Design review of the part built by this model. Coordinates are the model's own, in mm. Face numbers are marked on the shaded views. A direction names the side the tool comes from. Round coordinates to 2 decimals unless told otherwise and drop trailing zeros. Write item = value, one per line. Start each with the question number.
Item 1: Add section A-A, the plane x = 56. State how many separate pieces and enclosed holes the cut face has, then the cut area to 3 significant figures.
Item 2: For pin 1 Ø1 at (x, y) = (-46.5, 58) entering from +Z; pin 2 Ø1.5 at (x, z) = (-59.5, 37.5) entering from +Y; pin 3 Ø1.5 at (x, y) = (22, 33.5) entering from +Z; pin 4 Ø10 at (x, z) = (-12, -47) entering from +Y, all flat-tipped, find the tip position at first contact; note any pin that passes through.
Item 3: Machinability: for the marked faces 5 and 6, which of the approach directions +Z, -Z, +X, -X, +Y, -Y give a long, thin tool a straight path to every point of the face, cutting with its end or side? Answer none if there is none.
Item 4: To check wall thickness, follow L1, parallel to Y at x = 44, z = -19; L2, parallel to Z at x = -21.5, y = 62; L3, parallel to Z at x = -14, y = 57. State the ranges of each line that lie inside material, in increasing order.
Item 5: Mouldability with a two-part tool opening along Z and no side actions: class the marked faces 1, 2, 3 and 4 as released by +Z, released by -Z, zero draft, split by the parting line, or undercut.
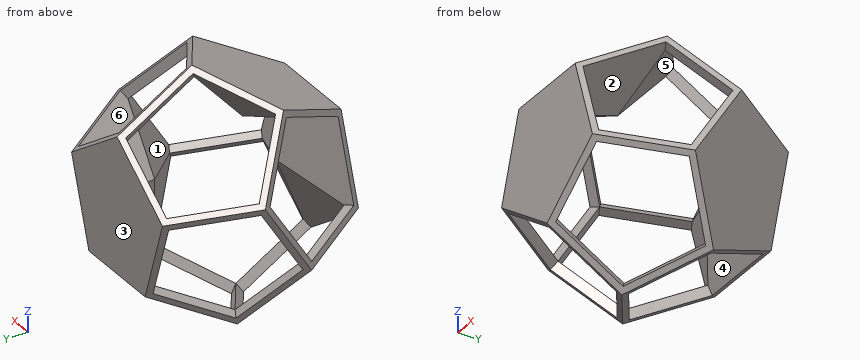
from build123d import *

# Parameters (mm, degrees)
CREATION_EXTRUDE_DEPTH = 130.901699304
CREATION_EXTRUDE_TAPER = -26.56505118
SKETCH2_OUTSIDE_W      = 455.432
SKETCH2_OUTSIDE_H      = 443.246
CREATION_CUT_DEPTH     = 130.901699304
CREATION_CUT_TAPER     = 26.56505118
CUT_EXTRUDE_B_DEPTH    = 50.8
C_INV_DEPTH            = 50.8
CUT_EXTRUDE_D_DEPTH    = 50.8
D_INV_DEPTH            = 50.8
CUT_EXTRUDE_E_DEPTH    = 50.8
E_INV_DEPTH            = 50.8
CUT_EXTRUDE_F_DEPTH    = 50.8
F_INV_DEPTH            = 50.8


with BuildPart() as part:
    # Sketch1 → creation_extrude (new body)
    with BuildSketch(Plane(origin=(0, 0, 0), x_dir=(1, 0, 0), z_dir=(0, 1, 0))):
        Polygon((0, 49.999999949), (-47.552825766, 15.450849703), (-29.389262585, -40.450849677), (29.389262585, -40.450849677), (47.552825766, 15.450849703), align=None)
    extrude(amount=CREATION_EXTRUDE_DEPTH, taper=CREATION_EXTRUDE_TAPER)

    # Sketch2 outside → creation_cut (cut)
    with BuildSketch(Plane(origin=(0, 130.901699304, 0), x_dir=(1, 0, 0), z_dir=(0, 1, 0))):
        with Locations((0, 12.5)):
            Rectangle(SKETCH2_OUTSIDE_W, SKETCH2_OUTSIDE_H)
        Polygon((0, -49.999999949), (47.552825766, -15.450849703), (29.389262585, 40.450849677), (-29.389262585, 40.450849677), (-47.552825766, -15.450849703), align=None, mode=Mode.SUBTRACT)
    extrude(amount=-CREATION_CUT_DEPTH, taper=CREATION_CUT_TAPER, mode=Mode.SUBTRACT)

    # Sketch5 → Cut-Extrude B (cut)
    with BuildSketch(Plane(origin=(0, 42.360679738, -84.721359466), x_dir=(-1, 0, 0), z_dir=(-9.08060963965006e-15, 0.4472135955455734, -0.8944271909771081))):
        Polygon((-42.797543189, 44.635254864), (1e-09, 13.541019643), (42.79754319, 44.635254866), (26.450336325, 94.946784308), (-26.450336327, 94.946784307), align=None)
    extrude(amount=-CUT_EXTRUDE_B_DEPTH, mode=Mode.SUBTRACT)

    # Sketch8 → C_inv (cut)
    with BuildSketch(Plane(origin=(-30.776835339, -16.180339872, 9.999999989), x_dir=(0.2446443083020028, 0.12861712429362696, 0.9610446387935747), z_dir=(-0.8506508083303469, -0.4472135955455736, 0.27639320224297786))):
        Polygon((-31.935023341, 77.848060657), (-22.992425992, 25.708717357), (29.358450763, 18.101689683), (52.77047459, 65.539631327), (14.889024305, 102.464919293), align=None)
    extrude(amount=-C_INV_DEPTH, mode=Mode.SUBTRACT)

    # Sketch9 → Cut-Extrude D (cut)
    with BuildSketch(Plane(origin=(49.797965648, 42.360679738, 68.541019594), x_dir=(0.8506508083603209, -0.27639320226847824, -0.44721359547279954), z_dir=(0.5257311121057348, 0.44721359554557366, 0.7236067977315217))):
        Polygon((-4.184405192, 98.473361345), (-54.495934634, 82.126154482), (-54.495934634, 29.22548183), (-4.184405192, 12.878274966), (26.90983003, 55.675818156), align=None)
    extrude(amount=-CUT_EXTRUDE_D_DEPTH, mode=Mode.SUBTRACT)

    # Sketch10 → D_inv (cut)
    with BuildSketch(Plane(origin=(-19.021130306, -16.180339872, -26.180339859), x_dir=(-0.8506508083603233, 0.27639320226847536, 0.44721359547279665), z_dir=(-0.5257311121057309, -0.44721359554557344, -0.7236067977315247))):
        Polygon((31.995934659, 98.473361351), (-18.315594783, 82.126154488), (-18.315594783, 29.225481836), (31.995934659, 12.878274972), (63.090169881, 55.675818162), align=None)
    extrude(amount=-D_INV_DEPTH, mode=Mode.SUBTRACT)

    # Sketch11 → Cut-Extrude E (cut)
    with BuildSketch(Plane(origin=(-49.797965648, 42.360679738, 68.541019594), x_dir=(0.8506508083603298, 0.2763932022684677, 0.447213595472789), z_dir=(-0.5257311121057203, 0.44721359554557355, 0.7236067977315324))):
        Polygon((4.184405192, 98.473361345), (-26.90983003, 55.675818156), (4.184405192, 12.878274966), (54.495934634, 29.22548183), (54.495934634, 82.126154482), align=None)
    extrude(amount=-CUT_EXTRUDE_E_DEPTH, mode=Mode.SUBTRACT)

    # Sketch12 → E_inv (cut)
    with BuildSketch(Plane(origin=(19.021130306, -16.180339872, -26.180339859), x_dir=(-0.8506508083603274, -0.27639320226847064, -0.44721359547279194), z_dir=(0.5257311121057243, -0.44721359554557355, -0.7236067977315294))):
        Polygon((-31.99593466, 98.473361351), (-63.090169881, 55.67581816), (-31.995934658, 12.878274972), (18.315594784, 29.225481837), (18.315594782, 82.126154489), align=None)
    extrude(amount=-E_INV_DEPTH, mode=Mode.SUBTRACT)

    # Sketch13 → Cut-Extrude F (cut)
    with BuildSketch(Plane(origin=(-80.574800989, 42.360679738, -26.180339862), x_dir=(-0.24464430830199108, 0.12861712429362016, 0.9610446387935785), z_dir=(-0.8506508083303513, 0.4472135955455735, -0.2763932022429644))):
        Polygon((-12.522250637, 97.763517637), (-35.934274461, 50.325575991), (1.947175826, 13.400288027), (48.771223471, 38.017146666), (39.828626119, 90.156489966), align=None)
    extrude(amount=-CUT_EXTRUDE_F_DEPTH, mode=Mode.SUBTRACT)

    # Sketch14 → F_inv (cut)
    with BuildSketch(Plane(origin=(30.776835339, -16.180339872, 9.999999989), x_dir=(0.2446443083019939, -0.12861712429362177, -0.9610446387935776), z_dir=(0.8506508083303502, -0.4472135955455736, 0.2763932022429676))):
        Polygon((-29.358450768, 18.101689686), (22.992425988, 25.708717353), (31.935023344, 77.848060652), (-14.889024299, 102.464919294), (-52.770474589, 65.539631333), align=None)
    extrude(amount=-F_INV_DEPTH, mode=Mode.SUBTRACT)


with BuildPart() as body_2:
    # of the pieces the cut leaves, the one that is kept (f_inv_keep)
    add(part.part.solids().sort_by_distance((0, 0, -49.999999949))[0])


solid = body_2.part
Result set:
q1.separate_pieces = 3
q1.enclosed_holes = 0
q1.area = 1,790 mm²
q2.pin_1 = through
q2.pin_2 = 69.71
q2.pin_3 = 57.58
q2.pin_4 = 127.8
q3.face_5 = none
q3.face_6 = +Z
q4.L1 = 1.57 to 4.13, 75.3 to 116.37
q4.L2 = -72.7 to -69.81, 61.99 to 71.45
q4.L3 = -75.06 to -72.39, 53.23 to 68.95
q5.face_1 = undercut
q5.face_2 = undercut
q5.face_3 = zero draft
q5.face_4 = released by -Z
